from build123d import *

# Parameters (mm, degrees)
SKETCH1_R           = 60
BOSS_EXTRUDE1_DEPTH = 25
BOSS_EXTRUDE2_DEPTH = 40
SKETCH3_W           = 80
SKETCH3_H           = 60
CUT_EXTRUDE1_DEPTH  = 60
SKETCH4_R           = 5
CUT_EXTRUDE2_DEPTH  = 5


with BuildPart() as part:
    # Sketch1 → Boss-Extrude1 (new body)
    with BuildSketch(Plane(origin=(0, 0, 0), x_dir=(1, 0, 0), z_dir=(0, 1, 0))):
        Circle(SKETCH1_R)
    extrude(amount=BOSS_EXTRUDE1_DEPTH)

    # Sketch2 → Boss-Extrude2 (add)
    with BuildSketch(Plane.XY):
        with BuildLine():
            Line((-40, 25), (0, 25))
            Line((0, 25), (40, 25))
            ThreePointArc((40, 25), (0, 65), (-40, 25))
        make_face()
    boss_extrude2 = extrude(amount=BOSS_EXTRUDE2_DEPTH)

    # Mirror1: Boss-Extrude2 across plane
    add(boss_extrude2.mirror(Plane(origin=(0, 0, 0), x_dir=(1, 0, 0), z_dir=(0, 0, -1))))

    # Sketch3 → Cut-Extrude1 (cut)
    with BuildSketch(Plane(origin=(0, 25, 0), x_dir=(1, 0, 0), z_dir=(0, 1, 0))):
        Rectangle(SKETCH3_W, SKETCH3_H)
    extrude(amount=CUT_EXTRUDE1_DEPTH, mode=Mode.SUBTRACT)

    # Sketch4 → Cut-Extrude2 (cut)
    with BuildSketch(Plane.XY.offset(-30)):
        with Locations((0, 55)):
            Circle(SKETCH4_R)
    cut_extrude2 = extrude(amount=-CUT_EXTRUDE2_DEPTH, mode=Mode.SUBTRACT)

    # Mirror2: Cut-Extrude2 across plane
    add(cut_extrude2.mirror(Plane(origin=(0, 0, 0), x_dir=(1, 0, 0), z_dir=(0, 0, -1))), mode=Mode.SUBTRACT)


solid = part.part
Could you check a few things on this model? Use its own coordinates, in mm. A direction names the side the tool comes from. Give positions to 0.01 mm unless a question says otherwise; leave off trailing zeros. Order: outer loops, then holes, each group sorted by start corner. A loop starts at its lowest first (then second) coordinate and runs counter-clockwise, first axis right, second up.
Item 1: If we section it at D-D, the plane y = 5: Write out the boundary of the cut face in (x, z).
Item 2: If we section it at B-B, the plane y = 35.5: Write out the boundary of the cut face in (x, z), plus the area to 3 significant figures.
Item 3: For faces 1 (the face through (-1, 40, 30)), 2 (the face through (0, 55, -35)), 3 (the face through (-1, 41, -40)), which set-ups out of +Z, -Z, +X, -X, +Y, -Y let a thin tool reach every point of the face, with its end or its side?
Item 4: I'm going to push flat-ended pins straight in: pin 1 (3 mm diameter, centred on x = -1, y = 54, fed in from +Z); pin 2 (4 mm diameter, centred on x = -39, z = -23.5, fed in from +Y); pin 3 (2 mm diameter, centred on y = 26.5, z = -23.5, fed in from +X); pin 4 (6 mm diameter, centred on x = 7.5, y = 49.5, fed in from -Z). Where does each tip first touch, or does it pass through?
Item 5: If we section it at C-C, the plane z = 32: Write out the boundary of the cut face in (x, y), plus the area to 3 significant figures.
Item 6: If we section it at A-A, the plane x = 0: Write out the boundary of the cut face in (y, z), plus the area to 3 significant figures.
Item 7: If we mould it in two halves opening along Z, with no side actions, what happens to faces 4 (the face through (0.88, 64.99, -34.93)), 5 (the face through (-1, 41, 40)), 6 (the face through (-1, 40, -30))? For each: pulls with the +Z half, pulls with the -Z half, needs draft (parallel to the pull), parting line crosses it, or undercut.
Item 8: I need wall thicknesses on line 1 (Y direction, x = 0, z = 33); line 2 (Z direction, x = 28, y = 29.5); line 3 (Y direction, x = -2.5, z = 51.5). Which ranges of each line are inside material? Lowest first, please.
Values:
1. outline: circle Ø120 at (0, 0)
2. outline: (-38.6, -40) - (38.6, -40) - (38.6, -30) - (-38.6, -30) - close; (-38.6, 30) - (38.6, 30) - (38.6, 40) - (-38.6, 40) - close
2. area: 1,540 mm2
3. face 1: +X, -X, +Y
3. face 2: none
3. face 3: -Z, +X, -X, +Y
4. pin 1: stops at z = 40
4. pin 2: stops at y = 25
4. pin 3: passes through
4. pin 4: stops at z = -40
5. outline: (-50.75, 0) - (50.75, 0) - (50.75, 25) - (40, 25) arc R40 ccw to (-40, 25) - (-50.75, 25) - close; hole circle Ø10 at (0, 55)
5. area: 4,970 mm2
6. outline: (0, -60) - (25, -60) - (25, -40) - (65, -40) - (65, -30) - (60, -30) - (60, -35) - (50, -35) - (50, -30) - (25, -30) - (25, 30) - (50, 30) - (50, 35) - (60, 35) - (60, 30) - (65, 30) - (65, 40) - (25, 40) - (25, 60) - (0, 60) - close
6. area: 3,700 mm2
7. face 4: needs draft
7. face 5: pulls with the +Z half
7. face 6: undercut
8. line 1: y = 0 to 50, 60 to 65
8. line 2: z = -40 to -30, 30 to 40
8. line 3: y = 0 to 25
